Geometry: see drawing. Coordinates: mm, zero at the bounding-box minimum. A direction names the side the tool comes from. Give positions to 0.01 mm unless a question says otherwise; leave off trailing zeros. Write each loop counter-clockwise with the first axis right and the second up, starting at its lowest first coordinate (ties: lowest second). Pieces come first, ordered by that corner, then holes. Notation, with made-up numbers: M -13.5,47.25 L -9.5,47.25 A30 cw -9.5,73.25 Z; hole C 66,85.25 d8. An arc over 180 degrees is marked long. Use a Markdown table: item, result. Add a question column.
1) Section C-C on x = 11. Return the cut outline in (y, z).
2) Section A-A on y = 25. Return the cut outline in (x, z).
3) Line query: line 1 (Y direction, x = 25, z = 6.5); line 2 (X direction, y = 44.5, z = 7); line 3 (X direction, y = 15.5, z = 9.75). Output: solid intervals per line, ascending.
4) Set-up query: the marked faces 4 and 5. Return all of +Z, -Z, +X, -X, +Y, -Y with unobstructed straight access to the full face (end or side cutting, diameter ignored); none if empty.
5) Draft query along Y for the marked faces 1, 2 and 3. Return one class per face: +Y half, -Y half, draft (parallel to the pull), parting line (faces both ways), or undercut.
6) Pin query (flat end, axial travel): pin 1 (4 mm diameter, centred on x = 43.5, y = 7.5, fed in from +Z); pin 2 (1.5 mm diameter, centred on x = 19.5, z = 4, fed in from -Y). Return the tip coordinate at first contact, or that it passes through.
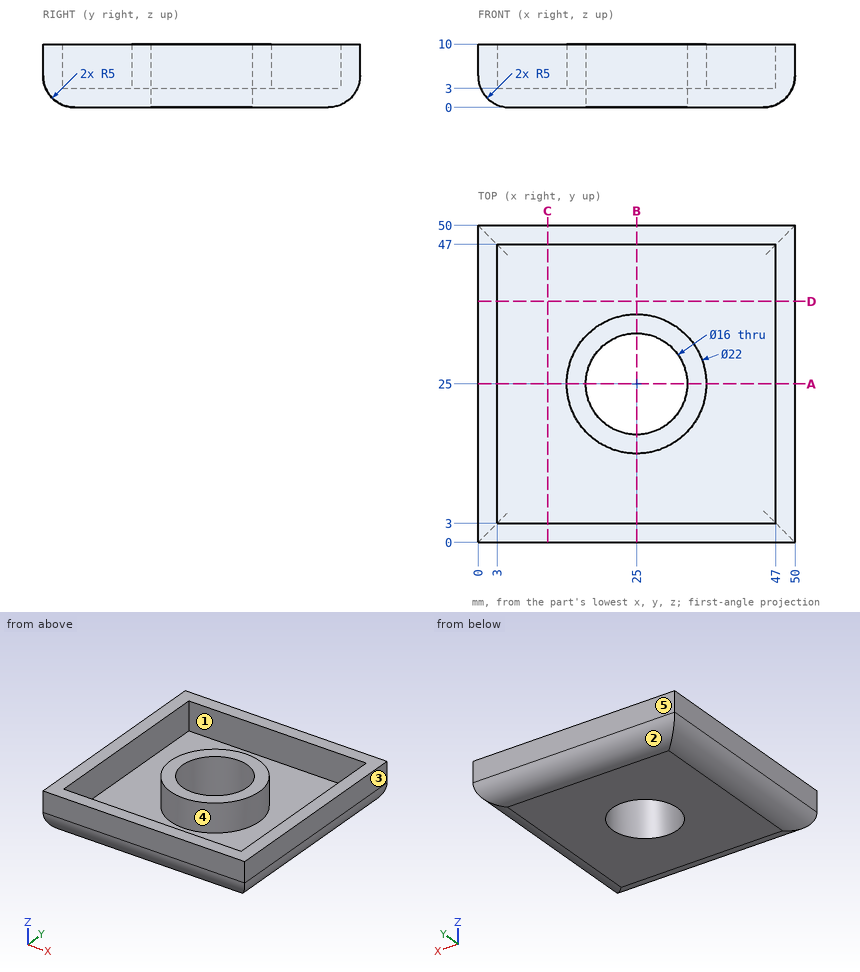
Found:
| question | item | result |
|---|---|---|
| 1 | outline | M 0,5 A5 ccw 5,0 L 45,0 A5 ccw 50,5 L 50,10 L 47,10 L 47,3 L 3,3 L 3,10 L 0,10 Z |
| 2 | outline | M 0,5 A5 ccw 5,0 L 17,0 L 17,10 L 14,10 L 14,3 L 3,3 L 3,10 L 0,10 Z; M 33,0 L 45,0 A5 ccw 50,5 L 50,10 L 47,10 L 47,3 L 36,3 L 36,10 L 33,10 Z |
| 3 | line 1 | 0 to 3, 14 to 17, 33 to 36, 47 to 50 |
| 3 | line 2 | 0 to 3, 47 to 50 |
| 3 | line 3 | 0 to 3, 19.45 to 30.55, 47 to 50 |
| 4 | face 4 | +Z |
| 4 | face 5 | +Z, -Z, +X, -X, +Y |
| 5 | face 1 | undercut |
| 5 | face 2 | +Y half |
| 5 | face 3 | draft |
| 6 | pin 1 | z = 3 |
| 6 | pin 2 | y = 0.01 |
